Check sheet for the modelled part. Datum: model origin and axes. Units: mm. Face numbers are marked on the shaded views. A direction names the side the tool comes from. Round coordinates to 2 decimals unless told otherwise and drop trailing zeros. Write each loop counter-clockwise with the first axis right and the second up, starting at its lowest first coordinate (ties: lowest second). Pieces come first, ordered by that corner, then holes. Notation, with made-up numbers: (4.25, 44.25) -> (8.25, 44.25) arc R22 cw to (8.25, 73.25) -> close; hole circle Ø5 at (-8, 16). An arc over 180 degrees is marked (long way). Put each result on its own line as item: value. Start each with the question number.
Autodesk Fusion 360 part; units mm, degrees
sketch "Sketch1" plane through (0, 0, 0) normal (0, 0, 1) x (1, 0, 0)
  line L0 (35, 45) -> (-35, 45)
  line L1 (-35, 45) -> (-35, -45)
  line L2 (-35, -45) -> (35, -45)
  line L3 (35, -45) -> (35, 45)
  line L4 (35, 45) -> (-35, -45) construction
  line L5 (-35, 45) -> (35, -45) construction
  line L6 (36, 46) -> (-36, 46)
  line L7 (-36, 46) -> (-36, -46)
  line L8 (-36, -46) -> (36, -46)
  line L9 (36, -46) -> (36, 46)
  line L10 (36, 46) -> (-36, -46) construction
  line L11 (-36, 46) -> (36, -46) construction
  dimension "d1" = 70
  dimension "d2" = 90
  dimension "d3" = 72
  dimension "d4" = 92
extrude "Extrude1" add sketch "Sketch1" along normal blind 1 contours L0 L1 L2 L3
extrude "Extrude2" add sketch "Sketch1" along normal blind 110
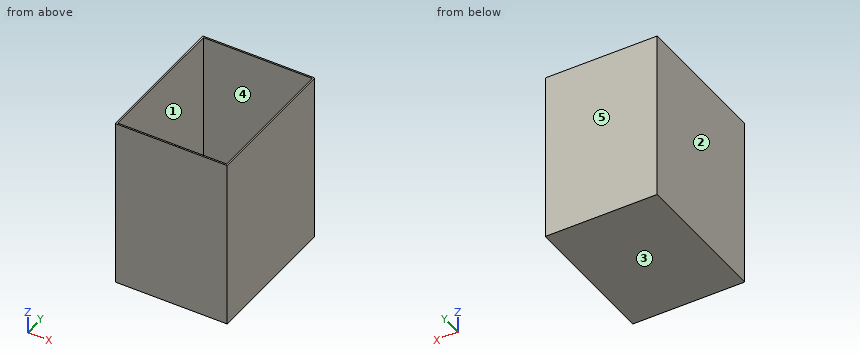
1. Section check A-A, the plane z = 28. Enter the section's corners in (x, y), then the cut area to 3 significant figures.
2. Section check B-B, the plane x = 9. Enter the section's corners in (y, z), then the cut area to 3 significant figures.
3. Access from +Z, -Z, +X, -X, +Y, -Y to the whole of each face (thin tool, end or side, straight path). Record for the marked faces 1 and 2.
4. Gauge pin test, flat end, axial feed: P1, Ø4, axis at x = 12.5, y = 1.5, coming from the +Z side. Record the tip position at first contact, or that the pin passes through.
5. Material ranges on L1, parallel to X at y = 9, z = 47; L2, parallel to Y at x = 7.5, z = 28.5; L3, parallel to Z at x = 15, y = -36, recorded low to high. Write a range as [from, to].
6. Section check C-C, the plane y = -13.5. Enter the section's corners in (x, z), then the cut area to 3 significant figures.
7. Draft check along Y on the marked faces 3, 4 and 5. Enter one of: released by +Y, released by -Y, zero draft, split by the parting line, or undercut.
Reply:
1. outline: (-36, -46) -> (36, -46) -> (36, 46) -> (-36, 46) -> close; hole (-35, -45) -> (35, -45) -> (35, 45) -> (-35, 45) -> close
1. area: 324 mm2
2. outline: (-46, 0) -> (46, 0) -> (46, 110) -> (45, 110) -> (45, 1) -> (-45, 1) -> (-45, 110) -> (-46, 110) -> close
2. area: 310 mm2
3. face 1: +Z
3. face 2: +Z, -Z, -X, +Y, -Y
4. P1: stops at z = 1
5. L1: x = [-36, -35], [35, 36]
5. L2: y = [-46, -45], [45, 46]
5. L3: z = [0, 1]
6. outline: (-36, 0) -> (36, 0) -> (36, 110) -> (35, 110) -> (35, 1) -> (-35, 1) -> (-35, 110) -> (-36, 110) -> close
6. area: 290 mm2
7. face 3: zero draft
7. face 4: undercut
7. face 5: released by +Y
